from build123d import *

# Parameters (mm, degrees)
SKETCH1_W           = 100
SKETCH1_H           = 26
BOSS_EXTRUDE1_DEPTH = 3
FILLET1_R           = 3


with BuildPart() as part:
    # Sketch1 → Boss-Extrude1 (new body)
    with BuildSketch(Plane.XY):
        with Locations((-69.498894811, -94.401018189)):
            Rectangle(SKETCH1_W, SKETCH1_H)
        with BuildLine():
            Line((-66.498894811, -88.401018189), (-66.498894811, -100.401018189))
            ThreePointArc((-66.498894811, -100.401018189), (-69.498894811, -103.401018189), (-72.498894811, -100.401018189))
            Line((-72.498894811, -100.401018189), (-72.498894811, -88.401018189))
            ThreePointArc((-72.498894811, -88.401018189), (-69.498894811, -85.401018189), (-66.498894811, -88.401018189))
        make_face(mode=Mode.SUBTRACT)
        with BuildLine():
            Line((-106.498894811, -88.401018189), (-106.498894811, -100.401018189))
            ThreePointArc((-106.498894811, -100.401018189), (-109.498894811, -103.401018189), (-112.498894811, -100.401018189))
            Line((-112.498894811, -100.401018189), (-112.498894811, -88.401018189))
            ThreePointArc((-112.498894811, -88.401018189), (-109.498894811, -85.401018189), (-106.498894811, -88.401018189))
        make_face(mode=Mode.SUBTRACT)
        with BuildLine():
            Line((-96.498894811, -88.401018189), (-96.498894811, -100.401018189))
            ThreePointArc((-96.498894811, -100.401018189), (-99.498894811, -103.401018189), (-102.498894811, -100.401018189))
            Line((-102.498894811, -100.401018189), (-102.498894811, -88.401018189))
            ThreePointArc((-102.498894811, -88.401018189), (-99.498894811, -85.401018189), (-96.498894811, -88.401018189))
        make_face(mode=Mode.SUBTRACT)
        with BuildLine():
            Line((-86.498894811, -88.401018189), (-86.498894811, -100.401018189))
            ThreePointArc((-86.498894811, -100.401018189), (-89.498894811, -103.401018189), (-92.498894811, -100.401018189))
            Line((-92.498894811, -100.401018189), (-92.498894811, -88.401018189))
            ThreePointArc((-92.498894811, -88.401018189), (-89.498894811, -85.401018189), (-86.498894811, -88.401018189))
        make_face(mode=Mode.SUBTRACT)
        with BuildLine():
            Line((-76.498894811, -88.401018189), (-76.498894811, -100.401018189))
            ThreePointArc((-76.498894811, -100.401018189), (-79.498894811, -103.401018189), (-82.498894811, -100.401018189))
            Line((-82.498894811, -100.401018189), (-82.498894811, -88.401018189))
            ThreePointArc((-82.498894811, -88.401018189), (-79.498894811, -85.401018189), (-76.498894811, -88.401018189))
        make_face(mode=Mode.SUBTRACT)
        with BuildLine():
            Line((-56.498894811, -88.401018189), (-56.498894811, -100.401018189))
            ThreePointArc((-56.498894811, -100.401018189), (-59.498894811, -103.401018189), (-62.498894811, -100.401018189))
            Line((-62.498894811, -100.401018189), (-62.498894811, -88.401018189))
            ThreePointArc((-62.498894811, -88.401018189), (-59.498894811, -85.401018189), (-56.498894811, -88.401018189))
        make_face(mode=Mode.SUBTRACT)
        with BuildLine():
            Line((-46.498894811, -88.355569142), (-46.498894811, -100.446467236))
            ThreePointArc((-46.498894811, -100.446467236), (-49.498894811, -103.446467236), (-52.498894811, -100.446467236))
            Line((-52.498894811, -100.446467236), (-52.498894811, -88.355569142))
            ThreePointArc((-52.498894811, -88.355569142), (-49.498894811, -85.355569142), (-46.498894811, -88.355569142))
        make_face(mode=Mode.SUBTRACT)
        with BuildLine():
            Line((-36.498894811, -88.346498653), (-36.498894811, -100.455537725))
            ThreePointArc((-36.498894811, -100.455537725), (-39.498894811, -103.455537725), (-42.498894811, -100.455537725))
            Line((-42.498894811, -100.455537725), (-42.498894811, -88.346498653))
            ThreePointArc((-42.498894811, -88.346498653), (-39.498894811, -85.346498653), (-36.498894811, -88.346498653))
        make_face(mode=Mode.SUBTRACT)
        with BuildLine():
            Line((-26.498894811, -88.531064652), (-26.498894811, -100.270971726))
            ThreePointArc((-26.498894811, -100.270971726), (-29.498894811, -103.270971726), (-32.498894811, -100.270971726))
            Line((-32.498894811, -100.270971726), (-32.498894811, -88.531064652))
            ThreePointArc((-32.498894811, -88.531064652), (-29.498894811, -85.531064652), (-26.498894811, -88.531064652))
        make_face(mode=Mode.SUBTRACT)
    extrude(amount=-BOSS_EXTRUDE1_DEPTH)

    # Fillet1
    fillet1_edges = [part.edges().sort_by_distance(p)[0] for p in [
        (-119.498894811, -81.401018189, -1.5),
        (-19.498894811, -81.401018189, -1.5),
        (-19.498894811, -107.401018189, -1.5),
        (-119.498894811, -107.401018189, -1.5),
    ]]
    fillet(fillet1_edges, radius=FILLET1_R)


solid = part.part
Model file for the job. Use its own axes, mm. A direction names the side the tool comes from. Give positions to 0.01 mm unless a question says otherwise; leave off trailing zeros. Write each loop counter-clockwise with the first axis right and the second up, starting at its lowest first coordinate (ties: lowest second). Pieces come first, ordered by that corner, then holes. Notation, with made-up numbers: M 76.5,39.25 L 91.5,39.25 A28 cw 91.5,71.25 Z; hole C 20,87.5 d1. An arc over 180 degrees is marked long. One line per item, written item: value. Start each with the question number.
Q1. Saw through at B-B, the plane y = -92.25. State how many separate pieces and enclosed holes the cut face has, plus the area to 3 significant figures.
Q2. Probe probe 1 along Y at (x, z) = (-39.5, -1.9); probe 2 along Y at (x, z) = (-89.5, -2.4); probe 3 along X at (y, z) = (-106, -2.15). List the from-to ranges inside material, lowest first. Write a range as [from, to].
Q3. Saw through at A-A, the plane x = -60. Write the cut outline in (y, z).
Q4. 3-axis set-ups, long thin cutter, end or side, ignore diameter. For faces 5 (the flat face through (-102.499, -94, -1)), 6 (the flat face through (-119.499, -95, -1)): which of +Z, -Z, +X, -X, +Y, -Y reach the whole face in a straight line?
Q5. Drop a flat-ended pin along its axis: pin 1 Ø8 at (x, y) = (-68, -97.5) entering from -Z. Give the stop position or say it passes through.
Q6. Saw through at D-D, the plane x = -31. Write the cut outline in (y, z), plus the area to 3 significant figures.
Q7. Two-plate mould, pull along Y, no slides. Class faces 1 (the cylindrical face through (-118.64, -82.3, -1.52)), 2 (the flat face through (-82.499, -94, -1)), 3 (the cylindrical face through (-118.64, -106.5, -1.52)), 4 (the flat face through (-81.3, -85.6, -3)): +Y half, -Y half, draft (parallel to the pull), parting line (faces both ways), or undercut.
Output values:
1. separate pieces: 10
1. enclosed holes: 0
1. area: 138 mm²
2. probe 1: y = [-107.4, -103.46], [-85.35, -81.4]
2. probe 2: y = [-107.4, -103.4], [-85.4, -81.4]
2. probe 3: x = [-119.04, -19.96]
3. outline: M -107.4,-3 L -103.36,-3 L -103.36,0 L -107.4,0 Z; M -85.44,-3 L -81.4,-3 L -81.4,0 L -85.44,0 Z
4. face 5: +Z, -Z
4. face 6: +Z, -Z, -X, +Y, -Y
5. pin 1: stops at z = -3
6. outline: M -107.4,-3 L -102.87,-3 L -102.87,0 L -107.4,0 Z; M -85.93,-3 L -81.4,-3 L -81.4,0 L -85.93,0 Z
6. area: 27.2 mm²
7. face 1: +Y half
7. face 2: undercut
7. face 3: -Y half
7. face 4: draft
